Design review of the part built by this model. Coordinates are the model's own, in mm. Round coordinates to 2 decimals unless told otherwise and drop trailing zeros. Loops run counter-clockwise (first coordinate to the right, second up) from the corner with the lowest first, then second, coordinate; pieces in that order, holes last. Notation, with made-up numbers: M 84.25,82.25 L 88.25,82.25 A29 ccw 88.25,120.25 Z; hole C 13,46.25 d5. An arc over 180 degrees is marked long. One line per item, written item: value. Start each with the question number.
Item 1: For line 1 along Y through (x, z) = (-3, 3.5); line 2 along X through (y, z) = (2.5, 3.5); line 3 along X through (y, z) = (1.5, 0.25), list the stretches that pass through material, from the lowest coordinate up.
Item 2: We need section C-C (z = -1). Write out the cut boundary in (x, y), then the cut area to 3 significant figures.
Item 3: Clearance check with flat-ended pins moving along their axes: pin 1 (2 mm diameter, centred on y = 5.5, z = -3.5, fed in from -X); pin 2 (5 mm diameter, centred on y = 0.5, z = 3.5, fed in from -X); pin 3 (6 mm diameter, centred on x = 6, z = -3, fed in from +Y). State where each tip first meets the part, or that it passes through.
Item 4: We need section B-B (x = 4.5). Write out the cut boundary in (y, z), then the cut area to 3 significant figures.
Item 5: We need section A-A (z = 4). Write out the cut boundary in (x, y).
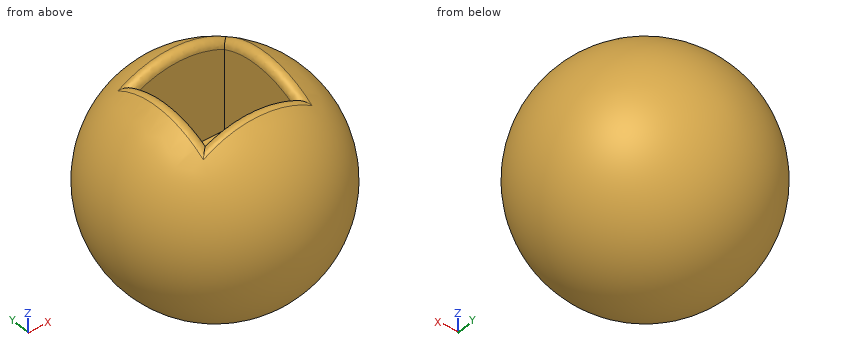
from build123d import *

# Parameters (mm, degrees)
SKETCH_2_W          = 6.2
SKETCH_2_H          = 6.2
CUT_EXTRUDE_1_DEPTH = 8
FILLET_1_R          = 0.5


with BuildPart() as part:
    # 스케치1 → 회전2 (revolve)
    with BuildSketch(Plane.XY):
        with BuildLine():
            Line((0, 8), (0, -8))
            ThreePointArc((0, -8), (8, 0), (0, 8))
        make_face()
    revolve(axis=Axis((0, 8, 0), (0, -1, 0)))

    # 스케치2 → 컷-돌출1 (cut)
    with BuildSketch(Plane.XY.offset(8)):
        Rectangle(SKETCH_2_W, SKETCH_2_H)
    extrude(amount=-CUT_EXTRUDE_1_DEPTH, mode=Mode.SUBTRACT)

    # 필렛1
    fillet_1_edges = [part.edges().sort_by_distance(p)[0] for p in [
        (0, -3.1, 7.374957627),
        (3.1, 0, 7.374957627),
        (0, 3.1, 7.374957627),
        (-3.1, 0, 7.374957627),
    ]]
    fillet(fillet_1_edges, radius=FILLET_1_R)


solid = part.part
A:
1. line 1: -6.54 to -3.1, 3.1 to 6.54
1. line 2: -6.75 to -3.1, 3.1 to 6.75
1. line 3: -7.85 to -3.1, 3.1 to 7.85
2. outline: C 0,0 d15.87
2. area: 198 mm2
3. pin 1: x = -5.79
3. pin 2: x = -7.93
3. pin 3: y = 7.09
4. outline: C 0,0 d13.23
4. area: 137 mm2
5. outline: C 0,0 d13.86; hole M -3.1,-3.1 L 3.1,-3.1 L 3.1,3.1 L -3.1,3.1 Z
